Check sheet for the modelled part. Datum: model origin and axes. Units: mm. A direction names the side the tool comes from. Give positions to 0.01 mm unless a question says otherwise; leave off trailing zeros. Loops run counter-clockwise (first coordinate to the right, second up) from the corner with the lowest first, then second, coordinate; pieces in that order, holes last. Notation, with made-up numbers: (31, 70.25) -> (78, 70.25) arc R28 ccw to (78, 88.25) -> close; hole circle Ø5 at (-8.5, -34). An arc over 180 degrees is marked (long way). Write each question's results on one line, items separated by ' | '. Start each with the question number.
1. Cross-section at A-A on x = -10. Record the boundary of the cut face in (y, z), and give its area (4 significant figures).
2. Mould release check, pull along Y, two halves, no side actions. Record for faces 4 (the face through (5, 79, 0)), 5 (the face through (-10.088, 128.002, -0.246)), 6 (the face through (-11.352, 18.526, -0.246)), 7 (the face through (1, 0, 1)): +Y half, -Y half, draft (parallel to the pull), parting line (faces both ways), or undercut.
3. Material ranges on L1, parallel to Y at x = -10, z = -0.25; L2, parallel to X at y = 20, z = -0.05; L3, parallel to X at y = 138.5, z = 1.5, recorded low to high. Write a range as from..to.
4. Cross-section at C-C on y = 90.5. Record the boundary of the cut face in (x, z), and give its area (3 significant figures).
5. Cross-section at B-B on y = 20. Record the boundary of the cut face in (x, z), and give its area (4 significant figures).
6. Cross-section at D-D on z = 2.25. Record the boundary of the cut face in (x, y), and give its area (3 significant figures).
7. Gauge pin test, flat ends, axial feed: pin 1 Ø2 at (y, z) = (45, 2) entering from +X; pin 2 Ø6 at (x, y) = (-13.5, 48) entering from +Z; pin 3 Ø6.5 at (x, y) = (-10, 130) entering from -Z. Record the tip position at first contact, or that the pin passes through.
8. Tool access check on faces 1 (the face through (2, 79, 3)), 2 (the face through (-10, 74, 0)), 3 (the face through (-6, 74, -2)). Record the directions out of +Z, -Z, +X, -X, +Y, -Y that give a thin tool (end or side, any length) a straight path to the whole face; none if there is none.
Autodesk Inventor part; units mm, degrees
ref_plane "YZ Plane" through (0, 0, 0) normal (1, 0, 0) x (0, 1, 0)
ref_plane "XZ Plane" through (0, 0, 0) normal (0, 1, 0) x (-1, 0, 0)
ref_plane "XY Plane" through (0, 0, 0) normal (0, 0, 1) x (1, 0, 0)
sketch "Sketch1" plane through (0, 0, 0) normal (0, 1, 0) x (-1, 0, 0)
  line L0 (0, 0) -> (0, 6.5)
  line L1 (0, 0) -> (20, 0)
  line L2 (-2, -2) -> (20, -2)
  line L3 (-2, 0) -> (-2, 6.5)
  line L4 (20, -2) -> (20, 0)
  line L5 (-2, 0) -> (-8.5, 0)
  line L6 (-8.5, -2) -> (-2, -2)
  line L7 (-8.5, 0) -> (-8.5, -2)
  line L8 (-2, 6.5) -> (0, 6.5)
  dimension "d2" = 20
  dimension "d3" = 2
  dimension "d5" = 2
  dimension "d30" = 6.5
  dimension "d33" = 6.5
extrude "Extrusion1" add sketch "Sketch1" along normal blind 40
sketch "Sketch2" plane through (0, 0, 0) normal (0, -1, 0) x (1, 0, 0)
  line L0 (2, 0) -> (8.5, 0)
  line L1 (8.5, 0) -> (8.5, 6.5)
  line L2 (8.5, 6.5) -> (2, 6.5)
  line L3 (2, 6.5) -> (2, 0)
  point P0 (0, 0)
  dimension "d10" = 6.5
  dimension "d11" = 6.5
extrude "Extrusion2" add sketch "Sketch2" against normal blind 10
move faces "Move1" translate (0, 110, 0) faces at (-3.8333, 40, -1.3333)
sketch "Sketch3" plane through (22, 0, -2) normal (0, 0, -1) x (-1, 0, 0)
  line L0 (42, 0) -> (42, 40)
  circle A0 centre (32, 20) radius 3.5
  circle A1 centre (32, 20) radius 2
  line L1 (32, 20) -> (42, 20)
  line L2 (42, 0) -> (42, 40)
  line L3 (32, 20) -> (32, 130)
  point P0 (22, 0)
  dimension "d15" = 7
  dimension "d18" = 4
  dimension "d32" = 10
  dimension "d37" = 110
hole "Hole1" at (-10, 20, -2) at (-10, 130, -2) direction (0, 0, 1) diameter 4 end through all countersink diameter 7 countersink angle 90
properties part number "3DPrintBracket_Tall" material "PC/ABS Plastic"
Geometry says:
1) outline: (0, -2) -> (16.5, -2) -> (18, -0.5) -> (18, 0) -> (0, 0) -> close; (22, -0.5) -> (23.5, -2) -> (126.5, -2) -> (128, -0.5) -> (128, 0) -> (22, 0) -> close; (132, -0.5) -> (133.5, -2) -> (150, -2) -> (150, 0) -> (132, 0) -> close | area: 279.5 mm^2
2) face 4: draft | face 5: undercut | face 6: undercut | face 7: -Y half
3) L1: 0..18, 22..128, 132..150 | L2: -20..-12, -8..8.5 | L3: 0..2
4) outline: (-20, -2) -> (8.5, -2) -> (8.5, 0) -> (2, 0) -> (2, 6.5) -> (0, 6.5) -> (0, 0) -> (-20, 0) -> close | area: 70.0 mm^2
5) outline: (-20, -2) -> (-13.5, -2) -> (-12, -0.5) -> (-12, 0) -> (-20, 0) -> close; (-8, -0.5) -> (-6.5, -2) -> (8.5, -2) -> (8.5, 0) -> (2, 0) -> (2, 6.5) -> (0, 6.5) -> (0, 0) -> (-8, 0) -> close | area: 59.75 mm^2
6) outline: (0, 0) -> (8.5, 0) -> (8.5, 10) -> (2, 10) -> (2, 150) -> (0, 150) -> close | area: 365 mm^2
7) pin 1: x = 2 | pin 2: z = 0 | pin 3: z = -1.75
8) face 1: +Z, +X, +Y | face 2: +Z, -X, +Y, -Y | face 3: -Z, +X, -X, +Y, -Y
